```python
from build123d import *

# Parameters (mm, degrees)
F0_W      = 50
F0_H      = 18.5
F1_DEPTH  = 32.75
F2_R      = 2
F2_W      = 30
F2_H      = 9
F3_DEPTH  = 4
F5_DEPTH  = 10
F6_DEPTH  = 4
F7_W      = 14
F7_H      = 14.5
F7_W_2    = 13
F7_H_2    = 7.5
F7_H_3    = 2.5
F8_DEPTH  = 16.5
F9_W      = 18.5
F9_H      = 4.5
F10_DEPTH = 4.5
F9_H_2    = 5.25
F11_DEPTH = 5


with BuildPart() as f1:
    # F0 (on Top) → F1 (new body, symmetric)
    with BuildSketch(Plane.XY):
        with Locations((25, 0)):
            Rectangle(F0_W, F0_H)
    extrude(amount=F1_DEPTH, both=True)

    # F2 (on face) → F3 (cut)
    with BuildSketch(Plane.XY.offset(32.75)):
        with Locations((10.5, 3.75)):
            Circle(F2_R)
        with Locations((39.5, 3.75)):
            Circle(F2_R)
        with Locations((25, -4.75)):
            Rectangle(F2_W, F2_H)
    extrude(amount=-F3_DEPTH, mode=Mode.SUBTRACT)

    # F4 (on face) → F5 (join)
    with BuildSketch(Plane(origin=(0, 0, -32.75), x_dir=(1, 0, 0), z_dir=(0, 0, -1))):
        with BuildLine():
            Line((43, 5.25), (7, 5.25))
            ThreePointArc((7, 5.25), (6.9364916731, 4.75), (6.75, 4.2817541634))
            Line((6.75, 4.2817541634), (6.75, -9.25))
            Line((6.75, -9.25), (43.25, -9.25))
            Line((43.25, -9.25), (43.25, 4.2817541634))
            ThreePointArc((43.25, 4.2817541634), (43.0635083269, 4.75), (43, 5.25))
        make_face()
    extrude(amount=F5_DEPTH)

    # F4 (on face) → F6 (cut)
    with BuildSketch(Plane(origin=(0, 0, -32.75), x_dir=(1, 0, 0), z_dir=(0, 0, -1))):
        with BuildLine():
            Line((6.75, 5.25), (7, 5.25))
            ThreePointArc((7, 5.25), (3.0635083269, 5.75), (6.75, 4.2817541634))
            Line((6.75, 4.2817541634), (6.75, 5.25))
        make_face()
        with BuildLine():
            ThreePointArc((47, 5.25), (45, 7.25), (43, 5.25))
            Line((43, 5.25), (43.25, 5.25))
            Line((43.25, 5.25), (43.25, 4.2817541634))
            ThreePointArc((43.25, 4.2817541634), (45.5, 3.3135083269), (47, 5.25))
        make_face()
    extrude(amount=-F6_DEPTH, mode=Mode.SUBTRACT)

    # F7 (on face) → F8 (cut)
    with BuildSketch(Plane.XZ.offset(9.25)):
        Polygon((18, 8.25), (6, 8.25), (6, -21.75), (40, -21.75), (40, 8.25), (32, 8.25), align=None)
        with Locations((25, 15.5)):
            Rectangle(F7_W, F7_H)
        with Locations((11.5, 26.5)):
            Rectangle(F7_W_2, F7_H_2)
        with Locations((25, 26.5)):
            Rectangle(F7_W, F7_H_2)
        with Locations((38.5, 26.5)):
            Rectangle(F7_W_2, F7_H_2)
        with Locations((25, 31.5)):
            Rectangle(F7_W, F7_H_3)
    extrude(amount=-F8_DEPTH, mode=Mode.SUBTRACT)

    # F9 (on face) → F10 (join)
    with BuildSketch(Plane(origin=(0, 0, 0), x_dir=(0, -1, 0), z_dir=(-1, 0, 0))):
        with Locations((0, 30.5)):
            Rectangle(F9_W, F9_H)
    extrude(amount=F10_DEPTH)

    # F9 (on face) → F11 (cut)
    with BuildSketch(Plane(origin=(0, 0, 0), x_dir=(0, -1, 0), z_dir=(-1, 0, 0))):
        with Locations((0, 2.625)):
            Rectangle(F9_W, F9_H_2)
    extrude(amount=-F11_DEPTH, mode=Mode.SUBTRACT)


solid = f1.part
```
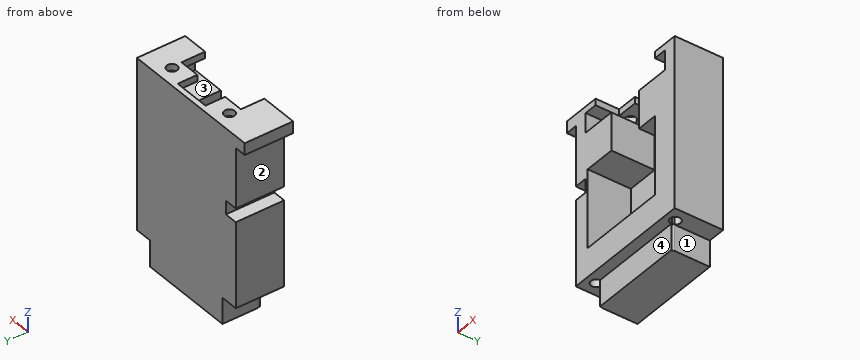
Model file for the job. Use its own axes, mm. Face numbers are marked on the shaded views. A direction names the side the tool comes from. Give positions to 0.01 mm unless a question says otherwise; leave off trailing zeros. Write each loop counter-clockwise with the first axis right and the second up, starting at its lowest first coordinate (ties: lowest second). Pieces come first, ordered by that corner, then holes. Notation, with made-up numbers: (4, 86.5) -> (14, 86.5) arc R19 ccw to (14, 90.5) -> close; hole circle Ø2 at (33, -3.5). An arc over 180 degrees is marked (long way). Use CSV: the item, a comma, the result in double quotes. Start each with the question number.
1) Drill centre lines: L1, parallel to Z at x = 15.5, y = 7; L2, parallel to Z at x = 3.5, y = 2.75; L3, parallel to Y at x = 5, z = -30. Where is each one in solid material? Low to high.
2) Tool access for the marked faces 1, 2, 3 and 4: list every direction of +Z, -Z, +X, -X, +Y, -Y with a clear straight run to the whole face (end or side of a thin tool).
3) Pin check, flat tips, straight feed: P1, Ø5, axis at y = -0.5, z = -3, coming from the -X side; P2, Ø1, axis at x = 31, y = 3.5, coming from the +Z side; P3, Ø3, axis at y = 1.5, z = -37.5, coming from the -X side. Stop position of each tip, or through.
4) Cut at A-A on z = 10. List the corners of the cut face in (x, y), plus the area to 3 significant figures.
5) Cut at B-B on x = 21.5. List the corners of the cut face in (y, z), plus the area to 4 significant figures.
6) Cut at C-C on y = 3.75. Count the separate pieces of the cut face and the enclosed holes in it, plus the area to 3 significant figures.
Final values:
1,L1,"z = -42.75 to -21.75, 8.25 to 22.75, 30.25 to 32.75"
1,L2,"z = -32.75 to 0, 5.25 to 32.75"
1,L3,"y = -9.25 to -7.25, -3.25 to 9.25"
2,face 1,"-Z, +X, +Y, -Y"
2,face 2,"-Z, -X, +Y, -Y"
2,face 3,"-Y"
2,face 4,"-Z, +X, -X, -Y"
3,P1,"stops at x = 0"
3,P2,"stops at z = -21.75"
3,P3,"stops at x = 6.75"
4,outline,"(0, -9.25) -> (18, -9.25) -> (18, 7.25) -> (32, 7.25) -> (32, -9.25) -> (50, -9.25) -> (50, 9.25) -> (0, 9.25) -> close"
4,area,"694 mm2"
5,outline,"(-9.25, -32.75) -> (-5.25, -32.75) -> (-5.25, -42.75) -> (9.25, -42.75) -> (9.25, 32.75) -> (7.25, 32.75) -> (7.25, -21.75) -> (-9.25, -21.75) -> close"
5,area,"457.5 mm2"
6,separate pieces,"3"
6,enclosed holes,"0"
6,area,"2,060 mm2"
